Could you check a few things on this drawing? It's one solid part, dimensions in mm from its lowest x, y, z. Give positions to 0.01 mm unless a question says otherwise; leave off trailing zeros. Loops run counter-clockwise (first coordinate to the right, second up) from the corner with the lowest first, then second, coordinate; pieces in that order, holes last. Notation, with made-up numbers: M 27.25,4 L 51.25,4 A9 ccw 51.25,15 Z; hole C 78.25,-29 d6. An arc over 180 degrees is marked long. Return JSON: item names as keys, results as strings. Group by question number.
1. If we section it at D-D (x = 32): Write out the boundary of the cut face in (y, z).
2. If we section it at C-C (z = 0.75): State how many separate pieces and enclosed holes the cut face has, plus the area to 3 significant figures.
3. If we section it at B-B (x = 38.5): Write out the boundary of the cut face in (y, z).
4. If we section it at A-A (y = 25): Write out the boundary of the cut face in (x, z).
5. For pin 1 (12 mm diameter, centred on x = 52.5, y = 53, fed in from +Z); pin 2 (1.5 mm diameter, centred on x = 36.5, z = 4, fed in from +Y); pin 3 (1.6 mm diameter, centred on x = 54.5, z = 3, fed in from +Y), each with a flat end and sliding along its axis, tell me the tip position at first contact or that it passes through.
6. Please list where these lines run through material, in increasing order: line 1 (Y direction, x = 40, z = 3.5); line 2 (Y direction, x = 49, z = 1.15).
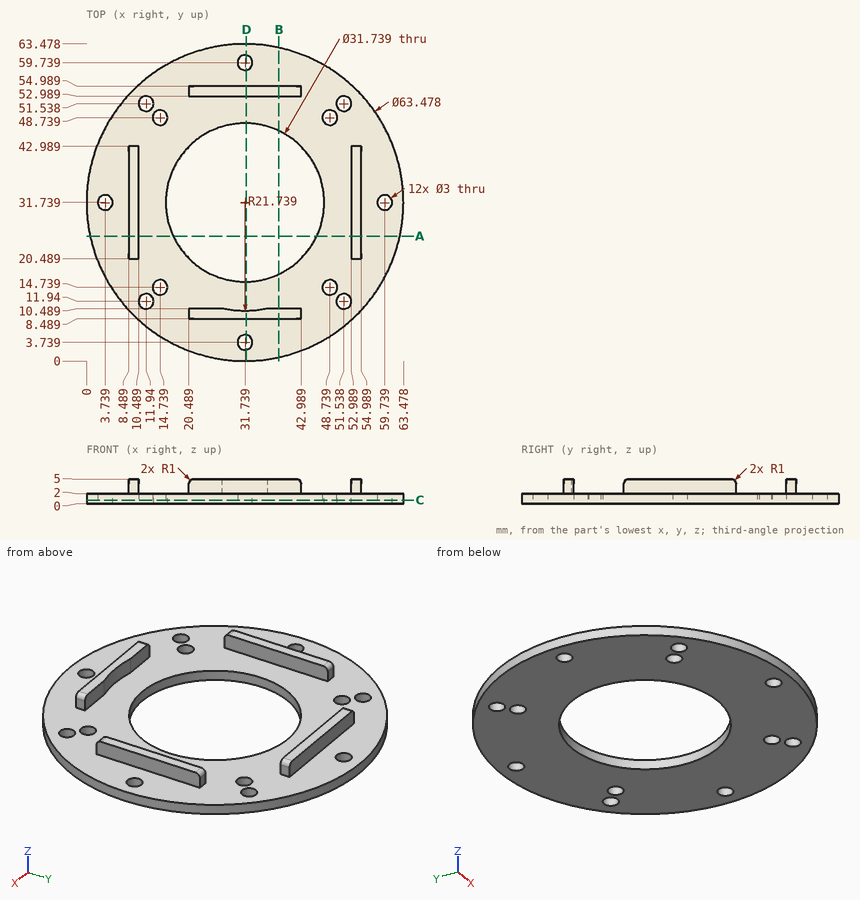
Answer:
{
 "1": {"outline": "M 0,0 L 2.26,0 L 2.26,2 L 0,2 Z; M 5.22,0 L 15.87,0 L 15.87,2 L 10,2 L 10,5 L 8.49,5 L 8.49,2 L 5.22,2 Z; M 47.61,0 L 58.26,0 L 58.26,2 L 54.99,2 L 54.99,5 L 52.99,5 L 52.99,2 L 47.61,2 Z; M 61.22,0 L 63.48,0 L 63.48,2 L 61.22,2 Z"},
 "2": {"separate pieces": "1", "enclosed holes": "13", "area": "2,290 mm²"},
 "3": {"outline": "M 0.73,0 L 17.38,0 L 17.38,2 L 10.49,2 L 10.49,5 L 8.49,5 L 8.49,2 L 0.73,2 Z; M 46.1,0 L 62.75,0 L 62.75,2 L 54.99,2 L 54.99,5 L 52.99,5 L 52.99,2 L 46.1,2 Z"},
 "4": {"outline": "M 0.72,0 L 17.37,0 L 17.37,2 L 10.49,2 L 10.49,5 L 8.49,5 L 8.49,2 L 0.72,2 Z; M 46.11,0 L 62.75,0 L 62.75,2 L 54.99,2 L 54.99,5 L 52.99,5 L 52.99,2 L 46.11,2 Z"},
 "5": {"pin 1": "stops at z = 2", "pin 2": "stops at y = 54.99", "pin 3": "stops at y = 42.99"},
 "6": {"line 1": "y = 8.49 to 10.49, 52.99 to 54.99", "line 2": "y = 5.1 to 13.26, 16.22 to 47.26, 50.22 to 58.37"}
}
